Read the model definition and answer for the solid it produces. Units are mm, in the model's axes. Face numbers are marked on the shaded views. A direction names the side the tool comes from. Coordinates: 2 decimals unless noted, no trailing zeros. Loops run counter-clockwise (first coordinate to the right, second up) from the corner with the lowest first, then second, coordinate; pieces in that order, holes last. Notation, with made-up numbers: M 36.5,84.25 L 91.5,84.25 A20 ccw 91.5,120.25 Z; hole C 13.25,23.25 d5. An arc over 180 degrees is marked long. Use one line per item in the form item = value. Start each with the question number.
1. Find the intervals of material crossed by probe 1 along Y at (x, z) = (-25.2, 0); probe 2 along X at (y, z) = (1.2, 8.25); probe 3 along X at (y, z) = (9, 2), in increasing order. Write a range as [from, to].
2. A tool of negligible diameter and unlimited length cuts with its end or side. For the marked faces 5, 6 and 7, from which of +Z, -Z, +X, -X, +Y, -Y can it reach the whole face along a straight path? Write none if from no direction.
3. The part is cut by section C-C (z = -8.5). Give the vertices of the cut face in (x, y).
4. The part is cut by section A-A (x = -9). Give the vertices of the cut face in (y, z).
5. For a pull along Z with two mould halves and no side action, classify the marked faces 1, 2, 3 and 4 as released by +Z, released by -Z, zero draft, split by the parting line, or undercut.
6. The part is cut by section D-D (x = 0). Give the vertices of the cut face in (y, z), plus the area to 3 significant figures.
7. Flat-ended cylindrical pins translate along their axes: pin 1 (6 mm diameter, centred on x = 18, z = 1, fed in from +Y); pin 2 (4.5 mm diameter, centred on x = -25.5, y = 17, fed in from +Z); pin 3 (3 mm diameter, centred on x = -24.5, y = 16.5, fed in from -Z); pin 4 (2 mm diameter, centred on x = 9, z = -8.25, fed in from +Y). Find the tip coordinate at first contact, or state that the pin passes through.
8. The part is cut by section B-B (y = 16.75). Give the vertices of the cut face in (x, z), plus the area to 3 significant figures.
from build123d import *

# Parameters (mm, degrees)
SKETCH1_W           = 54
SKETCH1_H           = 28.5
SKETCH1_W_2         = 5
SKETCH1_H_2         = 22.5
SKETCH1_R           = 1.7
SKETCH1_R_2         = 7.5
BOSS_EXTRUDE2_DEPTH = 3
SKETCH2_W           = 4
SKETCH2_H           = 20.5
BOSS_EXTRUDE3_DEPTH = 21.75
SKETCH4_R           = 10.25
BOSS_EXTRUDE4_DEPTH = 4
SKETCH6_R           = 4.4
SKETCH6_R_2         = 1.45
CUT_EXTRUDE3_DEPTH  = 4


with BuildPart() as part:
    # Sketch1 → Boss-Extrude2 (new body)
    with BuildSketch(Plane(origin=(0, 0, 0), x_dir=(1, 0, 0), z_dir=(0, 1, 0))):
        Rectangle(SKETCH1_W, SKETCH1_H)
        with Locations((20.5, 0)):
            Rectangle(SKETCH1_W_2, SKETCH1_H_2, mode=Mode.SUBTRACT)
        with Locations((-20.5, 0)):
            Rectangle(SKETCH1_W_2, SKETCH1_H_2, mode=Mode.SUBTRACT)
        with Locations(Location((-9, -8.25, 0), (0, 0, 270))):
            Circle(SKETCH1_R, mode=Mode.SUBTRACT)
        with Locations(Location((9, -8.25, 0), (0, 0, 270))):
            Circle(SKETCH1_R, mode=Mode.SUBTRACT)
        with Locations(Location((-9, 8.25, 0), (0, 0, 270))):
            Circle(SKETCH1_R, mode=Mode.SUBTRACT)
        with Locations(Location((0, 0, 0), (0, 0, 270))):
            Circle(SKETCH1_R_2, mode=Mode.SUBTRACT)
        with Locations(Location((9, 8.25, 0), (0, 0, 270))):
            Circle(SKETCH1_R, mode=Mode.SUBTRACT)
    extrude(amount=BOSS_EXTRUDE2_DEPTH)

    # Sketch2 → Boss-Extrude3 (add)
    with BuildSketch(Plane(origin=(0, 3, 0), x_dir=(1, 0, 0), z_dir=(0, 1, 0))):
        with Locations((25, 0)):
            Rectangle(SKETCH2_W, SKETCH2_H)
    boss_extrude3 = extrude(amount=BOSS_EXTRUDE3_DEPTH)

    # Sketch4 → Boss-Extrude4 (add)
    with BuildSketch(Plane(origin=(27, 0, 0), x_dir=(0, 0, -1), z_dir=(1, 0, 0))):
        with Locations((0, 24.75)):
            Circle(SKETCH4_R)
    boss_extrude4 = extrude(amount=-BOSS_EXTRUDE4_DEPTH)

    # Mirror1: Boss-Extrude3, Boss-Extrude4 across plane
    add(boss_extrude3.mirror(Plane(origin=(0, 0, 0), x_dir=(0, 0, 1), z_dir=(1, 0, 0))))
    add(boss_extrude4.mirror(Plane(origin=(0, 0, 0), x_dir=(0, 0, 1), z_dir=(1, 0, 0))))

    # Sketch6 → Cut-Extrude3 (cut)
    with BuildSketch(Plane(origin=(27, 0, 0), x_dir=(0, 0, -1), z_dir=(1, 0, 0))):
        with Locations((0, 24.75)):
            Circle(SKETCH6_R)
        with Locations((0, 32.75)):
            Circle(SKETCH6_R_2)
        with Locations((8, 24.75)):
            Circle(SKETCH6_R_2)
        with Locations((0, 16.75)):
            Circle(SKETCH6_R_2)
        with Locations((-8, 24.75)):
            Circle(SKETCH6_R_2)
    cut_extrude3 = extrude(amount=-CUT_EXTRUDE3_DEPTH, mode=Mode.SUBTRACT)

    # Mirror3: Cut-Extrude3 across plane
    add(cut_extrude3.mirror(Plane(origin=(0, 0, 0), x_dir=(0, 0, 1), z_dir=(1, 0, 0))), mode=Mode.SUBTRACT)


solid = part.part
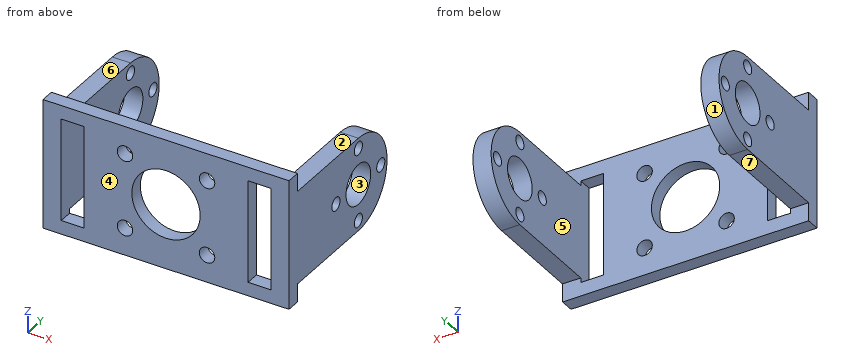
Computed values:
q1.probe_1 = [0, 15.3], [18.2, 20.35], [29.15, 31.3], [34.2, 35]
q1.probe_2 = [-27, -23], [-18, -10.7], [-7.3, 7.3], [10.7, 18], [23, 27]
q1.probe_3 = [-27, -23], [23, 27]
q2.face_5 = +Y, -Y
q2.face_6 = +Z, +X, -X, +Y
q2.face_7 = -Z, +X, -X, +Y
q3.outline = M -27,0 L -23,0 L -23,23.39 L -27,23.39 Z; M -27,26.11 L -23,26.11 L -23,30.48 L -27,30.48 Z; M -18,0 L -10.68,0 L -10.68,3 L -18,3 Z; M -7.32,0 L 7.32,0 L 7.32,3 L -7.32,3 Z; M 10.68,0 L 18,0 L 18,3 L 10.68,3 Z; M 23,0 L 27,0 L 27,23.39 L 23,23.39 Z; M 23,26.11 L 27,26.11 L 27,30.48 L 23,30.48 Z
q4.outline = M 0,-14.25 L 3,-14.25 L 3,-9.95 L 0,-9.95 Z; M 0,-6.55 L 3,-6.55 L 3,6.55 L 0,6.55 Z; M 0,9.95 L 3,9.95 L 3,14.25 L 0,14.25 Z
q5.face_1 = split by the parting line
q5.face_2 = released by +Z
q5.face_3 = undercut
q5.face_4 = zero draft
q6.outline = M 0,-14.25 L 3,-14.25 L 3,-7.5 L 0,-7.5 Z; M 0,7.5 L 3,7.5 L 3,14.25 L 0,14.25 Z
q6.area = 40.5 mm²
q7.pin_1 = 3
q7.pin_2 = 10.25
q7.pin_3 = -10.25
q7.pin_4 = through
q8.outline = M -27,-10.25 L -23,-10.25 L -23,-1.45 L -27,-1.45 Z; M -27,1.45 L -23,1.45 L -23,10.25 L -27,10.25 Z; M 23,-10.25 L 27,-10.25 L 27,-1.45 L 23,-1.45 Z; M 23,1.45 L 27,1.45 L 27,10.25 L 23,10.25 Z
q8.area = 141 mm²
